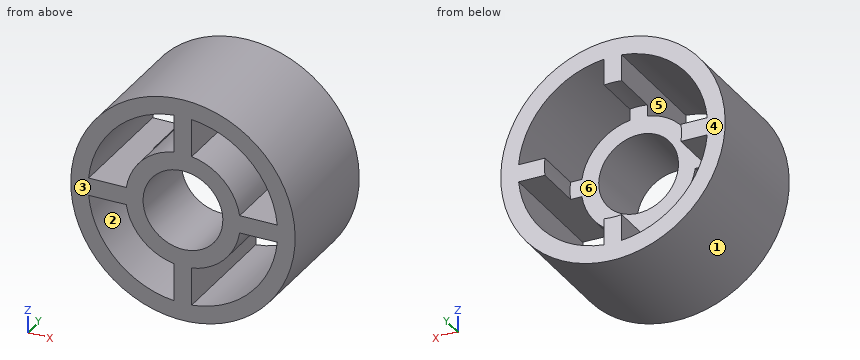
```python
from build123d import *

# Parameters (mm, degrees)
SKETCH_1_R          = 4.5
SKETCH_1_R_2        = 1.6
EXTRUDE_1_DEPTH     = 5
SKETCH_2_R          = 2.75
CUT_EXTRUDE_1_DEPTH = 2


with BuildPart() as part:
    # 草图1 → 凸台-拉伸1 (new body)
    with BuildSketch(Plane(origin=(0, 0, 0), x_dir=(1, 0, 0), z_dir=(0, 1, 0))):
        with Locations(Location((0, 0, 0), (0, 0, 270))):
            Circle(SKETCH_1_R)
        with Locations(Location((0, 0, 0), (0, 0, 270))):
            Circle(SKETCH_1_R_2, mode=Mode.SUBTRACT)
        with BuildLine():
            Line((2.273213584, 0.35), (3.783847249, 0.35))
            ThreePointArc((3.783847249, 0.35), (2.687005769, 2.687005769), (0.35, 3.783847249))
            Line((0.35, 3.783847249), (0.35, 2.273213584))
            ThreePointArc((0.35, 2.273213584), (1.626345597, 1.626345597), (2.273213584, 0.35))
        make_face(mode=Mode.SUBTRACT)
        with BuildLine():
            Line((2.273213584, -0.35), (3.783847249, -0.35))
            ThreePointArc((3.783847249, -0.35), (2.687005769, -2.687005769), (0.35, -3.783847249))
            Line((0.35, -3.783847249), (0.35, -2.273213584))
            ThreePointArc((0.35, -2.273213584), (1.626345597, -1.626345597), (2.273213584, -0.35))
        make_face(mode=Mode.SUBTRACT)
        with BuildLine():
            Line((-0.35, -2.273213584), (-0.35, -3.783847249))
            ThreePointArc((-0.35, -3.783847249), (-2.687005769, -2.687005769), (-3.783847249, -0.35))
            Line((-3.783847249, -0.35), (-2.273213584, -0.35))
            ThreePointArc((-2.273213584, -0.35), (-1.626345597, -1.626345597), (-0.35, -2.273213584))
        make_face(mode=Mode.SUBTRACT)
        with BuildLine():
            Line((-2.273213584, 0.35), (-3.783847249, 0.35))
            ThreePointArc((-3.783847249, 0.35), (-2.687005769, 2.687005769), (-0.35, 3.783847249))
            Line((-0.35, 3.783847249), (-0.35, 2.273213584))
            ThreePointArc((-0.35, 2.273213584), (-1.626345597, 1.626345597), (-2.273213584, 0.35))
        make_face(mode=Mode.SUBTRACT)
    extrude(amount=EXTRUDE_1_DEPTH)

    # 草图2 → 切除-拉伸1 (cut)
    with BuildSketch(Plane(origin=(0, 5, 0), x_dir=(1, 0, 0), z_dir=(0, 1, 0))):
        Circle(SKETCH_2_R)
    extrude(amount=-CUT_EXTRUDE_1_DEPTH, mode=Mode.SUBTRACT)


solid = part.part
```
Input: part model. Units: mm. Frame: model coordinates. Face numbers are marked on the shaded views. A direction names the side the tool comes from. Coordinates: 2 decimals unless noted, no trailing zeros. Loops run counter-clockwise (first coordinate to the right, second up) from the corner with the lowest first, then second, coordinate; pieces in that order, holes last. Notation, with made-up numbers: M 84,-20 L 123,-20 A28 cw 123,15 Z; hole C 27.25,-9 d9. An arc over 180 degrees is marked long. Use a Markdown table: item, result. Add a question column.
1) Section C-C, the plane y = 3.6. Return the cut outline in (x, z), plus the area to 3 significant figures.
2) Section A-A, the plane x = 0. Return the cut outline in (y, z).
3) Section B-B, the plane z = 0. Return the cut outline in (x, y), plus the area to 3 significant figures.
4) Pin query (flat end, axial travel): P1, Ø1.7, axis at x = 3.5, y = 1.5, coming from the -Z side; P2, Ø0.8, axis at x = -3.5, y = 2, coming from the +Z side; P3, Ø1.2, axis at y = 3.5, z = 3, coming from the -X side. Return the tip coordinate at first contact, or that it passes through.
5) Section D-D, the plane x = 3.5. Return the cut outline in (y, z).
6) Set-up query: the marked faces 4, 5 and 6. Return all of +Z, -Z, +X, -X, +Y, -Y with unobstructed straight access to the full face (end or side cutting, diameter ignored); none if empty.
7) Line query: L1, parallel to X at y = 1.3, z = 0; L2, parallel to Z at x = -3.5, y = 2.45; L3, parallel to Z at x = 1.75, y = 2.05. Output: solid intervals per line, ascending. Write a range as from..to.
8) Draft query along X for the marked faces 1, 2 and 3. Return one class per face: +X half, -X half, draft (parallel to the pull), parting line (faces both ways), or undercut.
Answer below:
| question | item | result |
|---|---|---|
| 1 | outline | C 0,0 d9; hole M -3.78,-0.35 A3.8 ccw -0.35,-3.78 L -0.35,-2.73 A2.75 ccw 0.35,-2.73 L 0.35,-3.78 A3.8 ccw 3.78,-0.35 L 2.73,-0.35 A2.75 ccw 2.73,0.35 L 3.78,0.35 A3.8 ccw 0.35,3.78 L 0.35,2.73 A2.75 ccw -0.35,2.73 L -0.35,3.78 A3.8 ccw -3.78,0.35 L -2.73,0.35 A2.75 ccw -2.73,-0.35 Z |
| 1 | area | 21.2 mm2 |
| 2 | outline | M 0,-4.5 L 5,-4.5 L 5,-2.75 L 3,-2.75 L 3,-1.6 L 0,-1.6 Z; M 0,1.6 L 3,1.6 L 3,2.75 L 5,2.75 L 5,4.5 L 0,4.5 Z |
| 3 | outline | M -4.5,0 L -1.6,0 L -1.6,3 L -2.75,3 L -2.75,5 L -4.5,5 Z; M 1.6,0 L 4.5,0 L 4.5,5 L 2.75,5 L 2.75,3 L 1.6,3 Z |
| 3 | area | 24.4 mm2 |
| 4 | P1 | z = -3.64 |
| 4 | P2 | z = 3.26 |
| 4 | P3 | x = -3.81 |
| 5 | outline | M 0,-2.83 L 5,-2.83 L 5,-1.48 L 0,-1.48 Z; M 0,-0.35 L 5,-0.35 L 5,0.35 L 0,0.35 Z; M 0,1.48 L 5,1.48 L 5,2.83 L 0,2.83 Z |
| 6 | face 4 | +Z, -Z, +X, -X, +Y |
| 6 | face 5 | +Y, -Y |
| 6 | face 6 | +Y |
| 7 | L1 | -4.5..-1.6, 1.6..4.5 |
| 7 | L2 | -2.83..-1.48, -0.35..0.35, 1.48..2.83 |
| 7 | L3 | -4.15..-3.37, -1.49..1.49, 3.37..4.15 |
| 8 | face 1 | parting line |
| 8 | face 2 | undercut |
| 8 | face 3 | draft |
